For this review, take the finished solid that the model builds, in its own axes (mm). Face numbers are marked on the shaded views. Coordinates: 2 decimals unless noted, no trailing zeros. Write each loop counter-clockwise with the first axis right and the second up, starting at its lowest first coordinate (ties: lowest second). Pieces come first, ordered by that corner, then holes. Notation, with made-up numbers: M 9,72 L 50,72 A28 cw 50,95 Z; hole C 87,77 d9. An arc over 180 degrees is marked long. One line per question, with ' | ' between items.
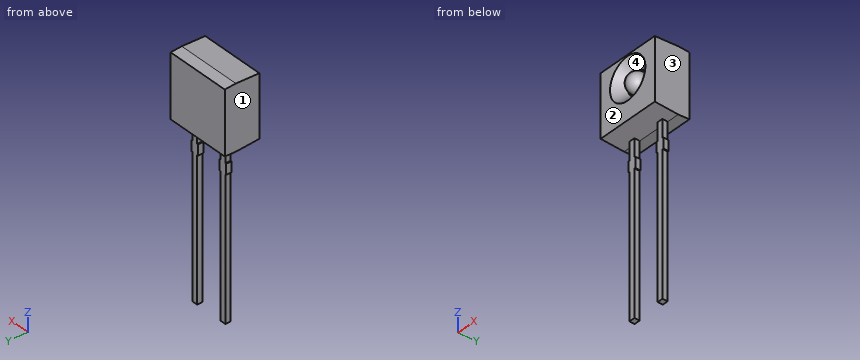
Autodesk Inventor part; units mm, degrees
ref_plane "YZ Plane" through (0, 0, 0) normal (1, 0, 0) x (0, 1, 0)
ref_plane "XZ Plane" through (0, 0, 0) normal (0, 1, 0) x (-1, 0, 0)
ref_plane "XY Plane" through (0, 0, 0) normal (0, 0, 1) x (1, 0, 0)
sketch "Skizze1" plane through (0, 0, 0) normal (1, 0, 0) x (0, 1, 0)
  line L0 (0.85, 1.755453) -> (0, 1.8)
  line L1 (0, 1.8) -> (-1.8, 1.705666)
  line L2 (-1.8, 1.705666) -> (-1.8, -3.005666)
  line L3 (-1.8, -3.005666) -> (0, -3.1)
  line L4 (0, -3.1) -> (0.85, -3.055453)
  line L5 (0.85, -3.055453) -> (0.85, 1.755453)
  line L6 (0, 2.78) -> (0, -4.08)
  line L7 (-2.33, 0) -> (1.38, 0)
  point P0 (0, 0)
  dimension "d0" = 2.65
  dimension "d1" = 4.9
  dimension "d2" = 3.1
  dimension "d3" = 3
  dimension "d4" = 3
  dimension "d5" = 3
  dimension "d6" = 3
  dimension "d7" = 1.8
sketch "Skizze1 outline for Extrusion1" plane through (0, 0, 0) normal (1, 0, 0) x (0, 1, 0)
  line L0 (0.85, 1.755453) -> (0, 1.8)
  line L1 (0, 1.8) -> (-1.8, 1.705666)
  line L2 (-1.8, 1.705666) -> (-1.8, -3.005666)
  line L3 (-1.8, -3.005666) -> (0, -3.1)
  line L4 (0, -3.1) -> (0.85, -3.055453)
  line L5 (0.85, -3.055453) -> (0.85, 1.755453)
extrude "Extrusion1" add sketch "Skizze1 outline for Extrusion1" along normal mid plane 4.9
sketch "Skizze2" plane through (0, 0, 0) normal (0, 1, 0) x (-1, 0, 0)
  line L0 (2.45, -3.1) -> (-2.45, -3.1)
  line L1 (1.495, -2.1) -> (1.045, -2.1)
  line L2 (1.045, -16) -> (1.495, -16)
  line L3 (0.97, -4.45) -> (0.97, -5.25)
  line L4 (1.57, -5.25) -> (1.57, -4.45)
  line L5 (1.57, -4.45) -> (1.495, -4.45)
  line L6 (1.045, -4.45) -> (0.97, -4.45)
  line L7 (1.495, -16) -> (1.495, -5.25)
  line L8 (1.495, -4.45) -> (1.495, -2.1)
  line L9 (1.045, -2.1) -> (1.045, -4.45)
  line L10 (1.045, -5.25) -> (1.045, -16)
  line L11 (0.97, -5.25) -> (1.045, -5.25)
  line L12 (1.495, -5.25) -> (1.57, -5.25)
  line L13 (1.27, -16) -> (1.27, -2.1) construction
  line L14 (2.45, 1.8) -> (-2.45, 1.8) construction
  line L15 (-2.45, 1.755453) -> (-2.45, 1.8) construction
  line L16 (2.45, 1.755453) -> (-2.45, 1.755453) construction
  line L17 (2.45, 1.8) -> (2.45, 1.755453) construction
  point P0 (0, 0)
  dimension "d10" = 0.45
  dimension "d11" = 0.6
  dimension "d12" = 0.8
  dimension "d13" = 2.15
  dimension "d14" = 1.27
  dimension "d15" = 17.8
  dimension "d16" = 1
sketch "Skizze2 outline for Extrusion2" plane through (0, 0, 0) normal (0, 1, 0) x (-1, 0, 0)
  line L0 (1.495, -4.45) -> (1.495, -2.1)
  line L1 (1.57, -4.45) -> (1.495, -4.45)
  line L2 (1.57, -5.25) -> (1.57, -4.45)
  line L3 (1.495, -5.25) -> (1.57, -5.25)
  line L4 (1.495, -16) -> (1.495, -5.25)
  line L5 (1.045, -16) -> (1.495, -16)
  line L6 (1.045, -5.25) -> (1.045, -16)
  line L7 (0.97, -5.25) -> (1.045, -5.25)
  line L8 (0.97, -4.45) -> (0.97, -5.25)
  line L9 (1.045, -4.45) -> (0.97, -4.45)
  line L10 (1.045, -2.1) -> (1.045, -4.45)
  line L11 (1.495, -2.1) -> (1.045, -2.1)
extrude "Extrusion2" add sketch "Skizze2 outline for Extrusion2" against normal blind 0.4
mirror "Spiegeln1" about plane through (0, 0, 0) normal (1, 0, 0) of "Extrusion2"
sketch "Skizze3" plane through (-2.45, -1.8, -3.005666) normal (0, -1, 0) x (1, 0, 0)
  line L0 (2.45, 5.785666) -> (2.45, -1.074334)
  line L1 (-0.98, 3.005666) -> (5.88, 3.005666)
  circle A0 centre (2.45, 3.005666) radius 1.6
  dimension "d19" = 3.2
sketch "Skizze3 outline for Extrusion3" plane through (-2.45, -1.8, -3.005666) normal (0, -1, 0) x (1, 0, 0)
  circle A0 centre (2.45, 3.005666) radius 1.6
extrude "Extrusion3" cut sketch "Skizze3 outline for Extrusion3" against normal blind 0.75 draft -45
sketch "Skizze4" plane through (0, 0, 0) normal (1, 0, 0) x (0, 1, 0)
  line L0 (-1.05, 0.85) -> (-1.05, -0.85)
  arc A0 (-1.05, 0.75) -> (-1.05, -0.75) centre (-1.05, 0) ccw
  line L1 (-2.371105, 0) -> (1.386851, 0)
  line L2 (-1.05, 0.75) -> (-1.05, -0.75)
  point P0 (0, 0)
  dimension "d22" = 0.75
sketch "Skizze4 outline for Umdrehung1" plane through (0, 0, 0) normal (1, 0, 0) x (0, 1, 0)
  line L0 (-1.05, -0.75) -> (-1.05, 0.75)
  arc A0 (-1.05, 0.75) -> (-1.05, -0.75) centre (-1.05, 0) ccw
revolve "Umdrehung1" add sketch "Skizze4 outline for Umdrehung1" angle 180 mid plane about axis through (0, -1.05, 0.75) along (0, 0, -1)
properties part number "IR Emitter TSKS5400S"
1) Insertion check: pin 1 Ø1.5 at (x, z) = (1, -8) entering from +Y; pin 2 Ø1 at (x, y) = (-2, -1.5) entering from -Z. Each pin has a flat end and moves straight along its axis. Give the tip position at first contact, or say it passes through.
Responses:
pin 1: y = 0 | pin 2: z = -3.05
2) The part is to be moulded in two halves that separate along X. For the marked faces 1, 2, 3 and 4, say which applies: +X half, -X half, draft (parallel to the pull), parting line (faces both ways), or undercut.
Responses:
face 1: -X half | face 2: draft | face 3: +X half | face 4: undercut
3) We need section A-A on z = -6.75. State the section outline as (x, y) points (3 decimals).
Responses:
outline: M -1.495,-0.4 L -1.045,-0.4 L -1.045,0 L -1.495,0 Z; M 1.045,-0.4 L 1.495,-0.4 L 1.495,0 L 1.045,0 Z
4) We need section C-C on z = 0. State the section outline as (x, y) points.
Responses:
outline: M -2.45,-1.8 L -1.6,-1.8 L -0.85,-1.05 L -0.75,-1.05 A0.75 ccw 0.75,-1.05 L 0.85,-1.05 L 1.6,-1.8 L 2.45,-1.8 L 2.45,0.85 L -2.45,0.85 Z
5) We need section D-D on x = 1.75. State the section outline as (y, z) points.
Responses:
outline: M -1.8,-3.01 L 0,-3.1 L 0.85,-3.06 L 0.85,1.76 L 0,1.8 L -1.8,1.71 Z
6) We need section B-B on x = 0. State the section outline as (y, z) points, then the cut area to 3 significant figures.
Responses:
outline: M -1.8,-3.01 L 0,-3.1 L 0.85,-3.06 L 0.85,1.76 L 0,1.8 L -1.8,1.71 L -1.8,1.6 L -1.05,0.85 L -1.05,0.75 A0.75 ccw -1.05,-0.75 L -1.05,-0.85 L -1.8,-1.6 Z | area: 11.8 mm^2
7) To check wall thickness, follow line 1 along X through (y, z) = (-0.05, -12.25) (3 decimals); line 2 along Y through (x, z) = (-1.3, -5.5); line 3 along Z through (x, y) = (-0.8, -1.5). State the ranges of each line that lie inside material, in increasing order. Write a range as [from, to].
Responses:
line 1: [-1.495, -1.045], [1.045, 1.495] | line 2: [-0.4, 0] | line 3: [-3.02, -1.02], [1.02, 1.72]
